Verification items for the finished model (mm, model axes). Face numbers are marked on the shaded views. A direction names the side the tool comes from. Give positions to 0.01 mm unless a question says otherwise; leave off trailing zeros. Loops run counter-clockwise (first coordinate to the right, second up) from the corner with the lowest first, then second, coordinate; pieces in that order, holes last. Notation, with made-up numbers: (60, -11) - (118, -11) arc R7 ccw to (118, 0) - close; hole circle Ø3 at (-32, 12.5). An arc over 180 degrees is marked (long way). One line per item, written item: value. Start each with the question number.
1. Mould release check, pull along Z, two halves, no side actions. Record for the marked faces 6, 7, 8 and 9: pulls with the +Z half, pulls with the -Z half, needs draft (parallel to the pull), parting line crosses it, or undercut.
2. Sectioned sample at D-D (z = 16.25). Record the cut outline in (x, y), plus the area to 3 significant figures.
3. Access from +Z, -Z, +X, -X, +Y, -Y to the whole of each face (thin tool, end or side, straight path). Record for the marked faces 1, 2, 3, 4 and 5.
4. Sectioned sample at B-B (z = 12). Record the cut outline in (x, y), plus the area to 3 significant figures.
5. Scan lines: L1, parallel to X at y = 14.5, z = 16.5; L2, parallel to X at y = 6, z = 12.25; L3, parallel to Y at x = 16.6, z = 2.7. Record each from-to range of solid material in increasing order. Write a range as [from, to].
6. Sectioned sample at C-C (y = 15.75). Record the cut outline in (x, z).
7. Gauge pin test, flat ends, axial feed: pin 1 (6.5 mm diameter, centred on x = 9, y = 6, fed in from +Z); pin 2 (1.6 mm diameter, centred on x = 23.5, z = 2.5, fed in from +Y); pin 3 (2.5 mm diameter, centred on x = 31.5, z = 9, fed in from +Y). Record the tip position at first contact, or that the pin passes through.
from build123d import *

# Parameters (mm, degrees)
EXTRUDE_1_DEPTH     = 3.2
EXTRUDE_2_DEPTH     = 2.6
EXTRUDE_3_DEPTH     = 3
CUT_EXTRUDE_1_DEPTH = 2.1
SKETCH_5_R          = 2.6
CUT_EXTRUDE_2_DEPTH = 1.1
CUT_EXTRUDE_3_DEPTH = 2.1
SKETCH_7_R          = 2.6
CUT_EXTRUDE_4_DEPTH = 0.9
SKETCH_8_R          = 2
CUT_EXTRUDE_5_DEPTH = 1.8


with BuildPart() as part:
    # ｽｹｯﾁ1 → ﾎﾞｽ - 押し出し1 (new body)
    with BuildSketch(Plane.XY):
        Polygon((0, 0), (13.621587752, 0), (19.578412248, 0), (33.2, 0), (33.2, 13.000240072), (19.578412248, 13.000240072), (13.621587752, 13.000240072), (0, 13.000240072), align=None)
    extrude(amount=EXTRUDE_1_DEPTH)

    # ｽｹｯﾁ2 → ﾎﾞｽ - 押し出し2 (add)
    with BuildSketch(Plane.ZY):
        with BuildLine():
            Line((3.199725342, 0), (15.472038891, 7.74466563))
            ThreePointArc((15.472038891, 7.74466563), (17.190896421, 14.371374104), (10.684882054, 16.501987504))
            Line((10.684882054, 16.501987504), (3.199725342, 13.000240072))
            Line((3.199725342, 13.000240072), (3.199725342, 0))
        make_face()
    extrude(amount=-EXTRUDE_2_DEPTH)

    # ｽｹｯﾁ3 → ﾎﾞｽ - 押し出し3 (add)
    with BuildSketch(Plane(origin=(33.2, 0, 0), x_dir=(0, 0, -1), z_dir=(1, 0, 0))):
        with BuildLine():
            Line((-3.199725342, 13.000240072), (-8.051923005, 17.315733546))
            ThreePointArc((-8.051923005, 17.315733546), (-18.828777882, 15.822754082), (-15.654913036, 5.416209475))
            Line((-15.654913036, 5.416209475), (-3.199725342, 0))
            Line((-3.199725342, 0), (-3.199725342, 13.000240072))
        make_face()
    extrude(amount=-EXTRUDE_3_DEPTH)

    # ｽｹｯﾁ4 → ｶｯﾄ - 押し出し1 (cut)
    with BuildSketch(Plane(origin=(0, 0, 0), x_dir=(-1, 0, 0), z_dir=(0, 0, -1))):
        with BuildLine():
            Line((-21.832955241, 8.023343606), (-20.309731671, 6.500120036))
            Line((-20.309731671, 6.500120036), (-21.832955241, 4.976896465))
            ThreePointArc((-21.832955241, 4.976896465), (-20.45383125, 2.646288786), (-18.12322357, 1.267164795))
            Line((-18.12322357, 1.267164795), (-16.6, 2.790388365))
            Line((-16.6, 2.790388365), (-15.07677643, 1.267164795))
            ThreePointArc((-15.07677643, 1.267164795), (-12.74616875, 2.646288786), (-11.367044759, 4.976896465))
            Line((-11.367044759, 4.976896465), (-12.890268329, 6.500120036))
            Line((-12.890268329, 6.500120036), (-11.367044759, 8.023343606))
            ThreePointArc((-11.367044759, 8.023343606), (-12.74616875, 10.353951285), (-15.07677643, 11.733075277))
            Line((-15.07677643, 11.733075277), (-16.6, 10.209851706))
            Line((-16.6, 10.209851706), (-18.12322357, 11.733075277))
            ThreePointArc((-18.12322357, 11.733075277), (-20.45383125, 10.353951285), (-21.832955241, 8.023343606))
        make_face()
    extrude(amount=-CUT_EXTRUDE_1_DEPTH, mode=Mode.SUBTRACT)

    # ｽｹｯﾁ5 → ｶｯﾄ - 押し出し2 (cut)
    with BuildSketch(Plane(origin=(0, 0, 2.1), x_dir=(-1, 0, 0), z_dir=(0, 0, -1))):
        with Locations((-16.6, 6.500120036)):
            Circle(SKETCH_5_R)
    extrude(amount=-CUT_EXTRUDE_2_DEPTH, mode=Mode.SUBTRACT)

    # ｽｹｯﾁ6 → ｶｯﾄ - 押し出し3 (cut)
    with BuildSketch(Plane.ZY.offset(-30.2)):
        with BuildLine():
            Line((15.503618238, 7.124116138), (15.503618238, 9.2730851))
            Line((15.503618238, 9.2730851), (17.6525872, 9.2730851))
            ThreePointArc((17.6525872, 9.2730851), (18.353618238, 11.9730851), (17.6525872, 14.6730851))
            Line((17.6525872, 14.6730851), (15.503618238, 14.6730851))
            Line((15.503618238, 14.6730851), (15.503618238, 16.822054063))
            ThreePointArc((15.503618238, 16.822054063), (12.803618238, 17.5230851), (10.103618238, 16.822054063))
            Line((10.103618238, 16.822054063), (10.103618238, 14.6730851))
            Line((10.103618238, 14.6730851), (7.954649275, 14.6730851))
            ThreePointArc((7.954649275, 14.6730851), (7.253618238, 11.9730851), (7.954649275, 9.2730851))
            Line((7.954649275, 9.2730851), (10.103618238, 9.2730851))
            Line((10.103618238, 9.2730851), (10.103618238, 7.124116138))
            ThreePointArc((10.103618238, 7.124116138), (12.803618238, 6.4230851), (15.503618238, 7.124116138))
        make_face()
    extrude(amount=-CUT_EXTRUDE_3_DEPTH, mode=Mode.SUBTRACT)

    # ｽｹｯﾁ7 → ｶｯﾄ - 押し出し4 (cut)
    with BuildSketch(Plane.ZY.offset(-32.3)):
        with Locations((12.803618238, 11.9730851)):
            Circle(SKETCH_7_R)
    extrude(amount=-CUT_EXTRUDE_4_DEPTH, mode=Mode.SUBTRACT)

    # ｽｹｯﾁ8 → ｶｯﾄ - 押し出し5 (cut)
    with BuildSketch(Plane(origin=(2.6, 0, 0), x_dir=(0, 0, -1), z_dir=(1, 0, 0))):
        with Locations((-12.803618238, 11.9730851)):
            Circle(SKETCH_8_R)
    extrude(amount=-CUT_EXTRUDE_5_DEPTH, mode=Mode.SUBTRACT)


solid = part.part
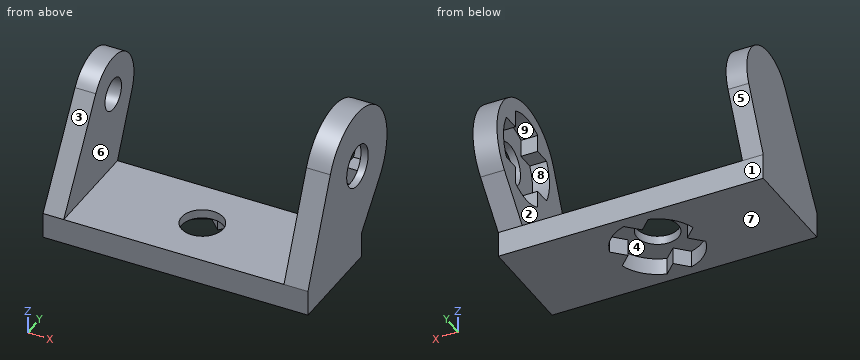
Results are:
1. face 6: needs draft
1. face 7: pulls with the -Z half
1. face 8: undercut
1. face 9: undercut
2. outline: (0, 8.35) - (2.6, 8.35) - (2.6, 15.6) - (0, 15.6) - close; (30.2, 5.71) - (33.2, 5.71) - (33.2, 18.24) - (30.2, 18.24) - (30.2, 14.67) - (32.3, 14.67) - (32.3, 9.27) - (30.2, 9.27) - close
2. area: 45.1 mm^2
3. face 1: -Z, +X, -X, +Y
3. face 2: +Z, +Y, -Y
3. face 3: +Z, -X, -Y
3. face 4: -Z
3. face 5: -Z, -X, +Y
4. outline: (0, 5.55) - (2.6, 5.55) - (2.6, 10.14) - (0.8, 10.14) - (0.8, 13.8) - (2.6, 13.8) - (2.6, 16.91) - (0, 16.91) - close; (30.2, 3.83) - (33.2, 3.83) - (33.2, 9.5) - (32.3, 9.5) - (32.3, 6.48) - (30.2, 6.48) - close; (30.2, 17.46) - (32.3, 17.46) - (32.3, 14.45) - (33.2, 14.45) - (33.2, 19.08) - (30.2, 19.08) - close
4. area: 41.2 mm^2
5. L1: x = [0, 2.6], [32.3, 33.2]
5. L2: x = [0, 2.6], [30.2, 33.2]
5. L3: y = [0, 3.9], [9.1, 13]
6. outline: (0, 9.08) - (2.6, 9.08) - (2.6, 16.08) - (0, 16.08) - close; (30.2, 6.29) - (33.2, 6.29) - (33.2, 18.87) - (30.2, 18.87) - (30.2, 15.5) - (32.3, 15.5) - (32.3, 10.1) - (30.2, 10.1) - close
7. pin 1: stops at z = 3.2
7. pin 2: stops at y = 13
7. pin 3: stops at y = 18.65
